CAD build for the part. Positions are in the model's coordinates, mm. Round coordinates to 2 decimals unless told otherwise and drop trailing zeros. Order: outer loops, then holes, each group sorted by start corner. A loop starts at its lowest first (then second) coordinate and runs counter-clockwise, first axis right, second up. Notation, with made-up numbers: (10, 8) - (61, 8) arc R19 cw to (61, 37) - close; hole circle Ø4 at (39.5, 14.5). An arc over 180 degrees is marked (long way). Use one line per item in the form item = value. Start each with the question number.
from build123d import *

# Parameters (mm, degrees)
F0_R     = 2.5
F1_DEPTH = 50


with BuildPart() as f1:
    # F0 (on Right) → F1 (new body)
    with BuildSketch(Plane.YZ):
        with BuildLine():
            Line((17.373618, -2), (4.582576, -2))
            ThreePointArc((4.582576, -2), (-2.738613, 4.1833), (0, -5))
            Line((0, -5), (17.373618, -5))
            Line((17.373618, -5), (17.373618, -2))
        make_face()
        Circle(F0_R, mode=Mode.SUBTRACT)
    extrude(amount=F1_DEPTH)


solid = f1.part
(1) Slice it at C-C (y = 1). Give the cut face in (x, z), and give its area (3 significant figures).
(2) Slice it at B-B (x = 35.5). Give the cut face in (y, z), and give its area (3 significant figures).
(3) Wall check: line 1 (Z direction, x = 30.5, y = 0); line 2 (Z direction, x = 17, y = 7.75); line 3 (Y direction, x = 35.5, z = -1.5). Give the ranges that are in metal, low to high. Write a range as [from, to].
(4) Mould opens along Y. For faces 1 (the flat face through (25, 17.374, -4)), 2 (the cylindrical face through (24.65, -0.54, -2.44)), 3 (the flat face through (50, 4, -1)) say: pulls with the +Y half, pulls with the -Y half, needs draft (parallel to the pull), parting line crosses it, or undercut.
(5) Slice it at D-D (y = 11.5). Give the cut face in (x, z).
(6) Slice it at A-A (z = 0). Give the cut face in (x, y).
(7) Flat gauge pins, fed straight in: P1, Ø10, axis at x = 34.5, y = 11, coming from the +Z side; P2, Ø3, axis at x = 6.5, z = 2, coming from the +Y side; P3, Ø5, axis at x = 10.5, z = -3.5, coming from the -Y side. Where does each tip first touch, or does it go through?
Results list:
q1.outline = (0, -5) - (50, -5) - (50, -2.29) - (0, -2.29) - close; (0, 2.29) - (50, 2.29) - (50, 4.9) - (0, 4.9) - close
q1.area = 266 mm²
q2.outline = (0, -5) - (17.37, -5) - (17.37, -2) - (4.58, -2) arc R5 ccw (long way) to start; hole circle Ø5 at (0, 0)
q2.area = 101 mm²
q3.line_1 = [-5, -2.5], [2.5, 5]
q3.line_2 = [-5, -2]
q3.line_3 = [-4.77, -2], [2, 4.77]
q4.face_1 = pulls with the +Y half
q4.face_2 = undercut
q4.face_3 = needs draft
q5.outline = (0, -5) - (50, -5) - (50, -2) - (0, -2) - close
q6.outline = (0, -5) - (50, -5) - (50, -2.5) - (0, -2.5) - close; (0, 2.5) - (50, 2.5) - (50, 5) - (0, 5) - close
q7.P1 = -2
q7.P2 = 4.97
q7.P3 = -4.9
